```python
from build123d import *

# Parameters (mm, degrees)
SKETCH1_R             = 20
BOSS_EXTRUDE1_DEPTH   = 4
SKETCH2_R             = 10
BOSS_EXTRUDE2_DEPTH   = 5
SKETCH4_R             = 3.975
BOSS_EXTRUDE3_DEPTH   = 10
M4_CLEARANCE_HOLE2_D  = 4.3
M3_TAPPED_HOLE1_D     = 2.5
M3_TAPPED_HOLE1_DEPTH = 5
M3_TAPPED_HOLE1_TIP   = 0.751075774
M3_TAPPED_HOLE2_D     = 2.5
M3_TAPPED_HOLE2_DEPTH = 5
M3_TAPPED_HOLE2_TIP   = 0.751075774


with BuildPart() as part:
    # Sketch1 → Boss-Extrude1 (new body)
    with BuildSketch(Plane(origin=(0, 0, 0), x_dir=(1, 0, 0), z_dir=(0, 1, 0))):
        with Locations(Location((0, 0, 0), (0, 0, 270))):
            Circle(SKETCH1_R)
    extrude(amount=BOSS_EXTRUDE1_DEPTH)

    # Sketch2 → Boss-Extrude2 (add)
    with BuildSketch(Plane(origin=(0, 4, 0), x_dir=(1, 0, 0), z_dir=(0, 1, 0))):
        with Locations(Location((0, 0, 0), (0, 0, 270))):
            Circle(SKETCH2_R)
    extrude(amount=BOSS_EXTRUDE2_DEPTH)

    # Sketch4 → Boss-Extrude3 (add)
    with BuildSketch(Plane(origin=(0, 9, 0), x_dir=(1, 0, 0), z_dir=(0, 1, 0))):
        with Locations(Location((0, 0, 0), (0, 0, 270))):
            Circle(SKETCH4_R)
    extrude(amount=BOSS_EXTRUDE3_DEPTH)

    # M4 Clearance Hole2 (through all)
    with Locations(Plane(origin=(0, 4, 0), x_dir=(1, 0, 0), z_dir=(0, 1, 0))):
        with Locations((-14, 0), (-7, 12.124355653), (7, 12.124355653), (14, 0), (7, -12.124355653), (-7, -12.124355653)):
            Hole(M4_CLEARANCE_HOLE2_D / 2)

    # M3 Tapped Hole1
    with Locations(Plane(origin=(0, 9, 0), x_dir=(1, 0, 0), z_dir=(0, 1, 0))):
        with Locations((-6.5, 0), (0, 6.5), (6.5, 0), (0, -6.5)):
            Hole(M3_TAPPED_HOLE1_D / 2, depth=M3_TAPPED_HOLE1_DEPTH)
            with Locations((0, 0, -(M3_TAPPED_HOLE1_DEPTH + M3_TAPPED_HOLE1_TIP / 2))):  # 118° drill point
                Cone(0, M3_TAPPED_HOLE1_D / 2, M3_TAPPED_HOLE1_TIP, mode=Mode.SUBTRACT)

    # M3 Tapped Hole2
    with Locations(Plane(origin=(0, 19, 0), x_dir=(1, 0, 0), z_dir=(0, 1, 0))):
        with Locations((0, 0)):
            Hole(M3_TAPPED_HOLE2_D / 2, depth=M3_TAPPED_HOLE2_DEPTH)
            with Locations((0, 0, -(M3_TAPPED_HOLE2_DEPTH + M3_TAPPED_HOLE2_TIP / 2))):  # 118° drill point
                Cone(0, M3_TAPPED_HOLE2_D / 2, M3_TAPPED_HOLE2_TIP, mode=Mode.SUBTRACT)


solid = part.part
```
Can you work these out from the model? Positions are in its coordinate system, mm. A direction names the side the tool comes from. Give positions to 0.01 mm unless a question says otherwise; leave off trailing zeros. Order: outer loops, then holes, each group sorted by start corner. A loop starts at its lowest first (then second) coordinate and runs counter-clockwise, first axis right, second up. Notation, with made-up numbers: (73, 57.25) - (90, 57.25) arc R25 ccw to (90, 92.25) - close; hole circle Ø1 at (18, 87.25). An arc over 180 degrees is marked (long way). Use a Markdown table: item, result. Add a question column.
Q1. If we section it at A-A on x = 14: Write out the boundary of the cut face in (y, z), plus the area to 3 significant figures.
Q2. If we section it at B-B on y = 15.25: Write out the boundary of the cut face in (x, z) (3 decimals), plus the area to 3 significant figures.
Q3. On a 3-axis mill with a long thin cutter (end or side, diameter ignored), from which of +Z, -Z, +X, -X, +Y, -Y can I reach the whole of each face in a straight line? I mean faces 1 (the cylindrical face through (7.75, 6.46, -0.05)), 2 (the cylindrical face through (-16.05, 1.97, -0.65)). Say none if no direction works.
Q4. Please list where these lines run through material, in increasing order: line 1 along Z through (x, y) = (14, 2.3); line 2 along Y through (x, z) = (-8, 16); line 3 along Z through (x, y) = (7, 2.2) (3 decimals).
Q5. If we section it at C-C on x = 2: Write out the boundary of the cut face in (y, z).
Q6. If we mould it in two halves opening along Z, with no side actions, what happens to faces 3 (the cylindrical face through (-19.524, 1.972, -4.336)), 4 (the cylindrical face through (7.466, 1.972, -10.025)), 5 (the flat face through (0.1, 9, 4.3)), 6 (the conical face through (-6.72, 3.38, -0.01))? For each: released by +Z, released by -Z, zero draft, split by the parting line, or undercut.
Q7. I'm going to push flat-ended pins straight in: pin 1 (1 mm diameter, centred on x = 13.5, z = -1, fed in from +Y); pin 2 (8 mm diameter, centred on x = -8, y = 12, fed in from +Z); pin 3 (7 mm diameter, centred on x = 7, z = -12.12, fed in from +Y); pin 4 (4 mm diameter, centred on x = 4, y = 4, fed in from -Z). Where does each tip first touch, or does it pass through?
Q8. If we section it at D-D on y = 11.5: Write out the boundary of the cut face in (x, z) (3 decimals), plus the area to 3 significant figures.
Answers follow:
| question | item | result |
|---|---|---|
| 1 | outline | (0, -14.28) - (4, -14.28) - (4, -2.15) - (0, -2.15) - close; (0, 2.15) - (4, 2.15) - (4, 14.28) - (0, 14.28) - close |
| 1 | area | 97.1 mm^2 |
| 2 | outline | circle Ø7.95 at (0, 0); hole circle Ø2.5 at (0, 0) |
| 2 | area | 44.7 mm^2 |
| 3 | face 1 | +Y |
| 3 | face 2 | +Y, -Y |
| 4 | line 1 | z = -14.28 to -2.15, 2.15 to 14.28 |
| 4 | line 2 | y = 0 to 4 |
| 4 | line 3 | z = -18.735 to -14.274, -9.974 to 9.974, 14.274 to 18.735 |
| 5 | outline | (0, -19.9) - (4, -19.9) - (4, -9.8) - (9, -9.8) - (9, -3.44) - (19, -3.44) - (19, 3.44) - (9, 3.44) - (9, 9.8) - (4, 9.8) - (4, 19.9) - (0, 19.9) - close |
| 6 | face 3 | split by the parting line |
| 6 | face 4 | undercut |
| 6 | face 5 | zero draft |
| 6 | face 6 | undercut |
| 7 | pin 1 | passes through |
| 7 | pin 2 | stops at z = 8.45 |
| 7 | pin 3 | stops at y = 4 |
| 7 | pin 4 | stops at z = -19.9 |
| 8 | outline | circle Ø7.95 at (0, 0) |
| 8 | area | 49.6 mm^2 |
